Read the model definition and answer for the solid it produces. Units are mm, in the model's axes. Face numbers are marked on the shaded views. Give positions to 0.01 mm unless a question says otherwise; leave off trailing zeros. Order: outer loops, then holes, each group sorted by start corner. A loop starts at its lowest first (then second) coordinate and runs counter-clockwise, first axis right, second up. Notation, with made-up numbers: (33, -28) - (75, -28) arc R25 ccw to (75, -16) - close; hole circle Ø11 at (-5, 18). An arc over 180 degrees is marked (long way). Return JSON: item names as keys, results as strings.
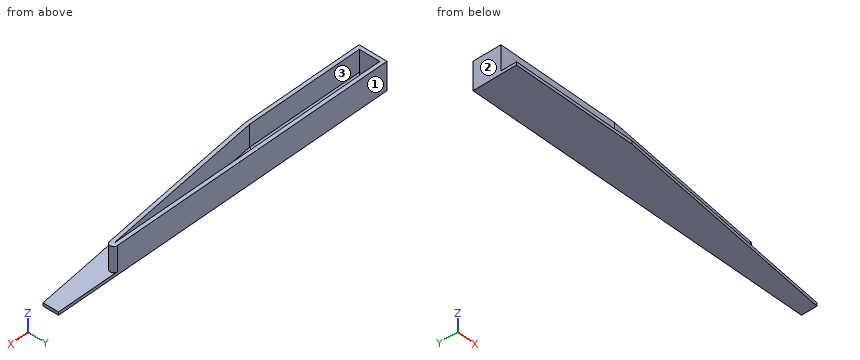
```python
from build123d import *

# Parameters (mm, degrees)
PAD_DEPTH                      = 1
PAD001_DEPTH                   = 8
CHAMFER_SIZE                   = 1
PART_MIRRORING_PLACEMENT_ANGLE = 180


with BuildPart() as body_ramp_support:
    # Sketch → Pad (new body)
    with BuildSketch(Plane.XY):
        Polygon((-40, 0), (-40, 14), (0, 14), (73.928571, 5), (73.928571, 0), align=None)
    extrude(amount=PAD_DEPTH)

    # Sketch001 (on Face7 of Pad) → Pad001 (join)
    with BuildSketch(Plane.XY.offset(1)):
        with BuildLine():
            Line((-40, 9), (-0.608696, 9))
            Line((-0.608696, 9), (53.677832, 2.391205))
            ThreePointArc((53.532815, 0), (54.730615, 1.127359), (53.677832, 2.391205))
            Line((-40, 0), (53.532815, 0))
            Line((-40, 0), (-40, 9))
        make_face()
        Polygon((53.532815, 1.2), (-0.753712, 7.808795), (-38.8, 7.808795), (-38.8, 1.2), align=None, mode=Mode.SUBTRACT)
    extrude(amount=PAD001_DEPTH)

    # Chamfer
    chamfer_edges = [body_ramp_support.edges().sort_by_distance(p)[0] for p in [
        (-19.776856, 7.808795, 1),
        (26.389552, 4.504397, 1),
        (7.366408, 1.2, 1),
        (-38.8, 4.504397, 1),
    ]]
    chamfer(chamfer_edges, length=CHAMFER_SIZE)


with BuildPart() as mirror_ramp_support:
    # Part__Mirroring: instance of Body-ramp-support
    add(body_ramp_support.part.mirror(Plane(origin=(0, 0, 0), x_dir=(0, -1, 0), z_dir=(1, 0, 0))))


with BuildPart() as mirror_ramp_support_1:
    # Part__Mirroring placement: moved
    add(mirror_ramp_support.part.moved(Location((0, -4, 0))).rotate(Axis((0, -4, 0), (0, 0, 1)), PART_MIRRORING_PLACEMENT_ANGLE))


solid = mirror_ramp_support_1.part
```
Q1. A cutting plane is placed at A-A (z = 4.5). Write down the section's boundary in (x, y).
Values:
{"outline": "(-40, -13) - (-0.61, -13) - (53.68, -6.39) arc R1.2 ccw to (53.53, -4) - (-40, -4) - close; hole (-38.8, -11.81) - (-0.75, -11.81) - (53.53, -5.2) - (-38.8, -5.2) - close"}
Q2. Determine the mould class of the marked faces 1, 2 and 3 for opening direction X: released by +X, released by -X, zero draft, split by the parting line, or undercut.
Values:
{"face 1": "zero draft", "face 2": "released by -X", "face 3": "undercut"}
Q3. A cutting plane is placed at D-D (x = 52.5). Write down the section's boundary in (y, z).
Values:
{"outline": "(-11.61, 0) - (-4, 0) - (-4, 9) - (-5.2, 9) - (-5.2, 2) - (-5.26, 1.94) - (-5.33, 2) - (-5.33, 9) - (-6.53, 9) - (-6.53, 1) - (-11.61, 1) - close"}
Q4. A cutting plane is placed at C-C (x = 27). Write down the section's boundary in (y, z), and give its area (3 significant figures).
Values:
{"outline": "(-14.71, 0) - (-4, 0) - (-4, 9) - (-5.2, 9) - (-5.2, 2) - (-6.2, 1) - (-7.42, 1) - (-8.43, 2) - (-8.43, 9) - (-9.64, 9) - (-9.64, 1) - (-14.71, 1) - close", "area": "31.0 mm²"}
Q5. Consider L1, parallel to Y at x = -6, z = 6.75; L2, parallel to Z at x = 53, y = -10; L3, parallel to Y at x = -16, z = 1.5. Determine where each line is inside the solid, lowest interval first.
Values:
{"L1": "y = -13 to -11.81, -5.2 to -4", "L2": "z = 0 to 1", "L3": "y = -13 to -11.31, -5.7 to -4"}
Q6. A cutting plane is placed at B-B (y = -7.5). Write down the section's boundary in (x, z).
Values:
{"outline": "(-40, 0) - (73.93, 0) - (73.93, 1) - (44.57, 1) - (44.57, 9) - (34.64, 9) - (34.64, 2) - (26.37, 1) - (-37.8, 1) - (-38.8, 2) - (-38.8, 9) - (-40, 9) - close"}
Q7. Given pin 1 (4 mm diameter, centred on x = 23.5, y = -13, fed in from +Z); pin 2 (1 mm diameter, centred on x = -2.5, y = -6, fed in from -Z); pin 3 (3.5 mm diameter, centred on y = -7, z = 7, fed in from +X); pin 4 (4 mm diameter, centred on x = -22, z = 6.5, fed in from -Y), each flat-ended and moving along its own axis, determine where each tip first touches the part or whether it passes through.
Values:
{"pin 1": "stops at z = 1", "pin 2": "stops at z = 0", "pin 3": "stops at x = 54.73", "pin 4": "stops at y = -13"}
